The model under review builds one solid part; all positions refer to its coordinate system, in mm. A direction names the side the tool comes from. Coordinates: 2 decimals unless noted, no trailing zeros. Loops run counter-clockwise (first coordinate to the right, second up) from the corner with the lowest first, then second, coordinate; pieces in that order, holes last. Notation, with made-up numbers: M 63.5,-18 L 114.5,-18 A26 ccw 114.5,13 Z; hole C 1.25,55.5 d4. An arc over 180 degrees is marked long. One line per item, written item: value.
```python
from build123d import *

# Parameters (mm, degrees)
BOX_W            = 120
BOX_H            = 80
BOX_DEPTH        = 15
POCKET_DEPTH     = 12
HOLE_D           = 4.5
HOLE_DEPTH       = 25
HOLE_CBORE_D     = 8
HOLE_CBORE_DEPTH = 4.4
SKETCH005_R      = 7.5
SKETCH005_W      = 13.5
SKETCH005_H      = 14.5
POCKET001_DEPTH  = 5


with BuildPart() as part:
    # Box → Box (join)
    with BuildSketch(Plane(origin=(-52.5, -46, 25), x_dir=(1, 0, 0), z_dir=(0, 0, 1))):
        with Locations((60, 40)):
            Rectangle(BOX_W, BOX_H)
    extrude(amount=BOX_DEPTH)

    # Sketch003 (on Face6 of Box) → Pocket (cut)
    with BuildSketch(Plane(origin=(-52.5, -46, 40), x_dir=(1, 0, 0), z_dir=(0, 0, 1))):
        with BuildLine():
            ThreePointArc((20, 75), (9.3933982822, 70.6066017178), (5, 60))
            Line((5, 20), (5, 60))
            ThreePointArc((5, 20), (9.3933982822, 9.3933982822), (20, 5))
            Line((100, 5), (20, 5))
            ThreePointArc((100, 5), (110.6066017178, 9.3933982822), (115, 20))
            Line((115, 60), (115, 20))
            ThreePointArc((115, 60), (110.6066017178, 70.6066017178), (100, 75))
            Line((20, 75), (100, 75))
        make_face()
    extrude(amount=-POCKET_DEPTH, mode=Mode.SUBTRACT)

    # Hole
    with Locations(Plane(origin=(-52.5, -46, 25), x_dir=(1, 0, 0), z_dir=(0, 0, -1))):
        with Locations((6, -6), (114, -6), (6, -74), (114, -74)):
            CounterBoreHole(HOLE_D / 2, HOLE_CBORE_D / 2, HOLE_CBORE_DEPTH, depth=HOLE_DEPTH)

    # Sketch005 (on Face5 of Hole) → Pocket001 (cut)
    with BuildSketch(Plane(origin=(-52.5, -46, 25), x_dir=(1, 0, 0), z_dir=(0, 0, -1))):
        with Locations((92.499962, -16.998899)):
            Circle(SKETCH005_R)
        with Locations((28.5389866751, -15.4398246124)):
            Rectangle(SKETCH005_W, SKETCH005_H)
    extrude(amount=-POCKET001_DEPTH, mode=Mode.SUBTRACT)


solid = part.part
```
(1) Add section D-D on x = 25.5. State the section outline as (y, z) points.
Checks:
outline: M -46,25 L 34,25 L 34,40 L 29,40 L 29,28 L -41,28 L -41,40 L -46,40 Z
(2) Draft analysis for pull direction Y (two halves, no side actions). For faces 1 (the face through (65.315, 26.799, 27.169)), 2 (the face through (63.286, 29.369, 34.774)), 3 (the face through (7, -46, 32)), 4 (the face through (7, -5, 25)), state which applies: pulls with the +Y half, pulls with the -Y half, needs draft (parallel to the pull), parting line crosses it, or undercut.
Checks:
face 1: undercut
face 2: undercut
face 3: pulls with the -Y half
face 4: needs draft
(3) Add section B-B on z = 34.5. State the section outline as (x, y) points, then the cut area to 3 significant figures.
Checks:
outline: M -52.5,-46 L 67.5,-46 L 67.5,34 L -52.5,34 Z; hole C -46.5,-40 d4.5; hole C -46.5,28 d4.5; hole M -47.5,-26 A15 ccw -32.5,-41 L 47.5,-41 A15 ccw 62.5,-26 L 62.5,14 A15 ccw 47.5,29 L -32.5,29 A15 ccw -47.5,14 Z; hole C 61.5,-40 d4.5; hole C 61.5,28 d4.5
area: 2,030 mm^2
(4) Add section A-A on x = -29. State the section outline as (y, z) points, then the cut area to 4 significant figures.
Checks:
outline: M -46,25 L -37.81,25 L -37.81,28 L -41,28 L -41,40 L -46,40 Z; M -23.31,25 L 34,25 L 34,40 L 29,40 L 29,28 L -23.31,28 Z
area: 316.5 mm^2
(5) Insertion check: pin 1 Ø10 at (x, y) = (2, -11) entering from +Z; pin 2 Ø7 at (x, y) = (-46.5, -40) entering from -Z; pin 3 Ø4 at (x, y) = (63.5, -38.5) entering from -Z. Each pin has a flat end and moves straight along its axis. Give the tip position at first contact, or say it passes through.
Checks:
pin 1: z = 28
pin 2: z = 29.4
pin 3: z = 25
(6) To check wall thickness, follow L1, parallel to Y at x = 61.5, z = 27.45; L2, parallel to Y at x = 7, z = 37.25; L3, parallel to Y at x = -44.5, z = 31.25. State the ranges of each line that lie inside material, in increasing order. Write a range as [from, to].
Checks:
L1: [-46, -44], [-36, 24], [32, 34]
L2: [-46, -41], [29, 34]
L3: [-46, -41.03], [-38.97, -35], [23, 26.97], [29.03, 34]
(7) Tool access review of faces 5 (the face through (-24, -37.81, 26)), 6 (the face through (8, -41, 34)), 7 (the face through (-49.45, -42.7, 27.17)): name each direction out of +Z, -Z, +X, -X, +Y, -Y from which nothing blocks a thin tool from reaching the whole face with its end or side.
Checks:
face 5: +Z, -Z
face 6: +Z
face 7: -Z
(8) Add section C-C on y = -33.5. State the section outline as (x, z) points.
Checks:
outline: M -52.5,25 L -30.71,25 L -30.71,28 L -45.49,28 L -45.49,40 L -52.5,40 Z; M -17.21,25 L 34,25 L 34,28 L -17.21,28 Z; M 46,25 L 67.5,25 L 67.5,40 L 60.49,40 L 60.49,28 L 46,28 Z
